The model under review builds one solid part; all positions refer to its coordinate system, in mm. Coordinates: 2 decimals unless noted, no trailing zeros. Order: outer loops, then holes, each group sorted by start corner. A loop starts at its lowest first (then second) coordinate and runs counter-clockwise, first axis right, second up.
from build123d import *

# Parameters (mm, degrees)
SKETCH1_W           = 63.8
SKETCH1_H           = 123.8
BOSS_EXTRUDE1_DEPTH = 3
SKETCH2_R           = 2
CUT_EXTRUDE1_DEPTH  = 70.700932562
FILLET1_R           = 6


with BuildPart() as part:
    # Sketch1 → Boss-Extrude1 (new body)
    with BuildSketch(Plane(origin=(0, 0, 0), x_dir=(1, 0, 0), z_dir=(0, 1, 0))):
        Rectangle(SKETCH1_W, SKETCH1_H)
    extrude(amount=BOSS_EXTRUDE1_DEPTH)

    # Sketch2 → Cut-Extrude1 (cut, through all)
    with BuildSketch(Plane(origin=(0, 3, 0), x_dir=(1, 0, 0), z_dir=(0, 1, 0))):
        with Locations(Location((0, -56.1, 0), (0, 0, 270))):
            Circle(SKETCH2_R)
    cut_extrude1 = extrude(amount=-CUT_EXTRUDE1_DEPTH, mode=Mode.SUBTRACT)

    # Sketch3 → CSK for M4 Hex Socket Countersunk Head Screw1 (revolve, cut)
    with BuildSketch(Plane(origin=(0, 0, 56.1), x_dir=(0, 0, -1), z_dir=(1, 0, 0))):
        Polygon((0, 0), (0, 3), (2, 3), (2, 2), (4, 0), align=None)
    csk_for_m4_hex_socket_countersunk_head_s = revolve(axis=Axis((0, -6.35, 56.1), (0, 1, 0)), mode=Mode.SUBTRACT)

    # Mirror1: Cut-Extrude1, CSK for M4 Hex Socket Countersunk Head Screw1 across plane
    add(cut_extrude1.mirror(Plane.XY), mode=Mode.SUBTRACT)
    add(csk_for_m4_hex_socket_countersunk_head_s.mirror(Plane.XY), mode=Mode.SUBTRACT)

    # Fillet1
    fillet1_edges = [part.edges().sort_by_distance(p)[0] for p in [
        (31.9, 1.5, 61.9),
        (-31.9, 1.5, 61.9),
        (-31.9, 1.5, -61.9),
        (31.9, 1.5, -61.9),
    ]]
    fillet(fillet1_edges, radius=FILLET1_R)


solid = part.part
(1) Insertion check: pin 1 Ø4.5 at (x, z) = (0, -56.1) entering from -Y. The pin has a flat end and moves straight along its axis. Give the tip position at first contact, or say it passes through.
(2) Wall thickness on line 1 (Z direction, x = 0, y = 2.5); line 2 (X direction, y = 2.8, z = 56.1); line 3 (X direction, y = 1.2, z = -54): over which ranges is each line inside the solid? List them lowest first.
(3) Consider section A-A (x = 0). Give the boundary of the cut face in (y, z), then the cut area to 3 significant figures.
(4) The part is to be moulded in two halves that separate along X. For faces 1 (the face through (0.088, 2.507, -54.102)), 2 (the face through (0, 3, -1)), 3 (the face through (-31.9, 1, 1)), say which applies: +X half, -X half, draft (parallel to the pull), parting line (faces both ways), or undercut.
Findings:
1. pin 1: stops at y = 1.75
2. line 1: z = -61.9 to -58.1, -54.1 to 54.1, 58.1 to 61.9
2. line 2: x = -31.9 to -2, 2 to 31.9
2. line 3: x = -31.9 to -1.85, 1.85 to 31.9
3. outline: (0, -61.9) - (3, -61.9) - (3, -58.1) - (2, -58.1) - (0, -60.1) - close; (0, -52.1) - (2, -54.1) - (3, -54.1) - (3, 54.1) - (2, 54.1) - (0, 52.1) - close; (0, 60.1) - (2, 58.1) - (3, 58.1) - (3, 61.9) - (0, 61.9) - close
3. area: 339 mm2
4. face 1: undercut
4. face 2: draft
4. face 3: -X half
